Print and shaded views of the part. All mm, measured from the part's lowest x, y and z. A direction names the side the tool comes from. Coordinates: 2 decimals unless noted, no trailing zeros. Return JSON: item names as keys, results as strings.
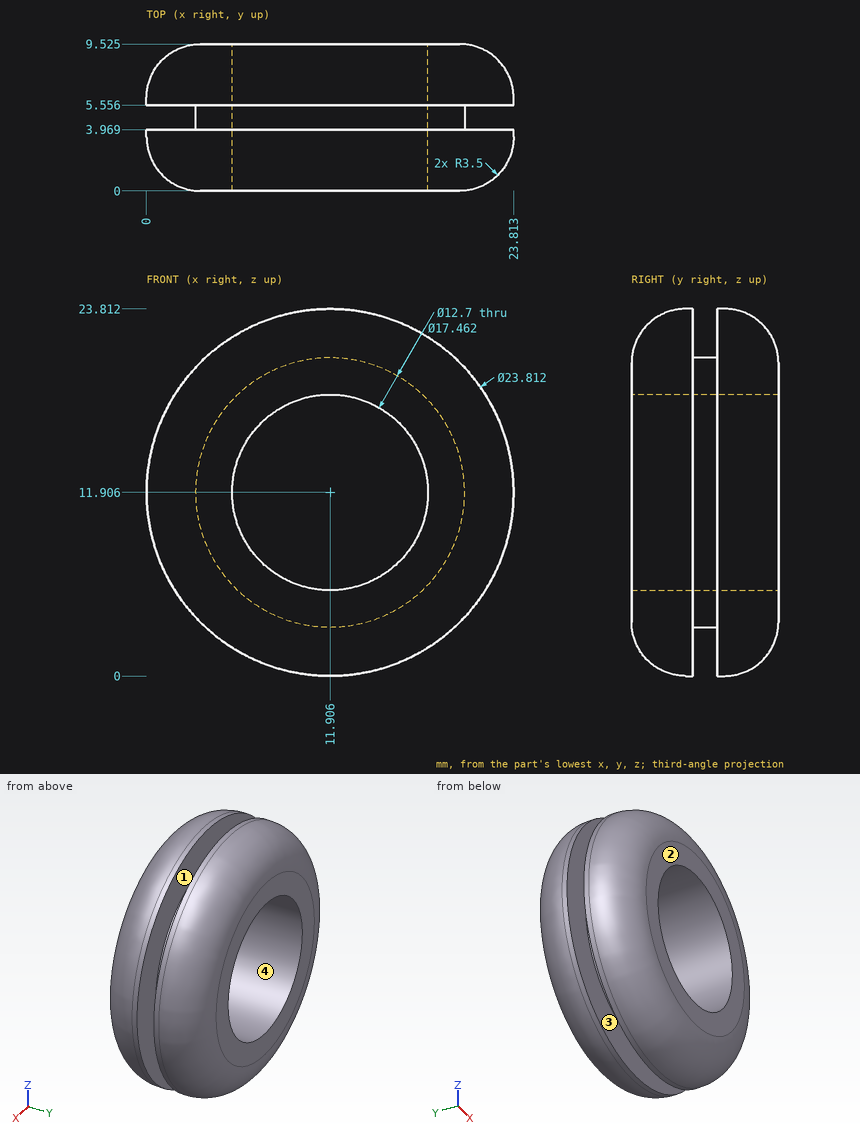
Item 1: Drop a flat-ended pin along its axis: pin 1 Ø1 at (x, y) = (9.5, 5) entering from -Z (1 decimal). Give the stop position or say it passes through.
Check result:
{"pin 1": "stops at z = 3.4"}
Item 2: Pull direction Z, two halves, no side cores. Call the marked faces 3 and 4: +Z half, -Z half, draft (parallel to the pull), parting line (faces both ways), or undercut.
Check result:
{"face 3": "draft", "face 4": "undercut"}
Item 3: 3-axis set-ups, long thin cutter, end or side, ignore diameter. For the marked faces 1 and 2: which of +Z, -Z, +X, -X, +Y, -Y reach the whole face in a straight line?
Check result:
{"face 1": "none", "face 2": "+Z, -Z, +X, -X, -Y"}
Item 4: Wall check: line 1 (X direction, y = 4.5, z = 13.25); line 2 (X direction, y = 2, z = 16.5) (1 decimal); line 3 (Y direction, x = 13, z = 1.75) (1 decimal). Give the ranges that are in metal, low to high.
Check result:
{"line 1": "x = 3.28 to 5.7, 18.11 to 20.53", "line 2": "x = 1.3 to 7.5, 16.3 to 22.5", "line 3": "y = 0.5 to 4, 5.6 to 9"}
